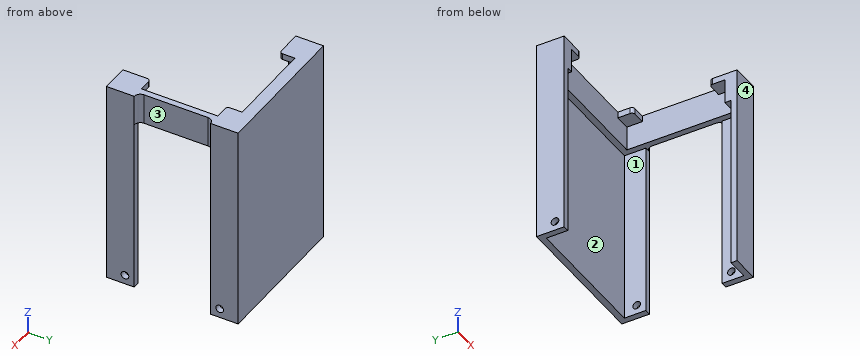
```python
from build123d import *

# Parameters (mm, degrees)
EXTRUDE_THIN1_DEPTH  = 10
SKETCH2_W            = 7
SKETCH2_H            = 7
BOSS_EXTRUDE1_DEPTH  = 2
FILLET1_R            = 1
BOSS_EXTRUDE2_DEPTH  = 67
SKETCH4_R            = 1.25
CUT_EXTRUDE1_DEPTH   = 91.624775862
FILLET2_R            = 2
MOVE_START           = -67
MOVE_FACE1_OUTLINE_W = 29.1
MOVE_FACE1_OUTLINE_H = 2
MOVE_FACE1_DEPTH     = 67


# Read off the part's stored shape, not the designer's step: Move Face1
with BuildPart() as part:
    # Sketch1 → Extrude-Thin1 (new body)
    with BuildSketch(Plane.XY):
        Polygon((0, -5), (0, 0), (39.1, 0), (39.1, -34.8), (34.1, -34.8), (34.1, -36.8), (41.1, -36.8), (41.1, 2), (-2, 2), (-2, -5), align=None)
    extrude(amount=-EXTRUDE_THIN1_DEPTH)

    # Sketch2 → Boss-Extrude1 (add)
    with BuildSketch(Plane.XY):
        with Locations((1.5, -1.5)):
            Rectangle(SKETCH2_W, SKETCH2_H)
        with Locations((37.6, -1.5)):
            Rectangle(SKETCH2_W, SKETCH2_H)
        with Locations((37.6, -33.3)):
            Rectangle(SKETCH2_W, SKETCH2_H)
    extrude(amount=-BOSS_EXTRUDE1_DEPTH)

    # Fillet1
    fillet1_edges = [part.edges().sort_by_distance(p)[0] for p in [
        (5, -5, -1),
        (34.1, -5, -1),
        (34.1, -29.8, -1),
    ]]
    fillet(fillet1_edges, radius=FILLET1_R)

    # Sketch3 → Boss-Extrude2 (add)
    with BuildSketch(Plane.XY):
        Polygon((34.1, 2), (41.1, 2), (41.1, -5), (43.1, -5), (43.1, 4), (34.1, 4), align=None)
    boss_extrude2 = extrude(amount=-BOSS_EXTRUDE2_DEPTH)

    # Mirror1: Boss-Extrude2 across plane
    add(boss_extrude2.mirror(Plane(origin=(19.55, 0, 0), x_dir=(0, 0, 1), z_dir=(1, 0, 0))))

    # Mirror2: Boss-Extrude2 across plane
    add(boss_extrude2.mirror(Plane.ZX.offset(-17.4)))

    # Sketch4 → Cut-Extrude1 (cut, through all)
    with BuildSketch(Plane(origin=(43.1, 0, 0), x_dir=(0, 0, -1), z_dir=(1, 0, 0))):
        with Locations((64, -2)):
            Circle(SKETCH4_R)
    cut_extrude1 = extrude(amount=-CUT_EXTRUDE1_DEPTH, mode=Mode.SUBTRACT)

    # Mirror3: Cut-Extrude1 across plane
    add(cut_extrude1.mirror(Plane.ZX.offset(-17.4)), mode=Mode.SUBTRACT)

    # Fillet2
    fillet2_edges = [part.edges().sort_by_distance(p)[0] for p in [
        (41.1, -29.8, -5),
        (41.1, -5, -5),
    ]]
    fillet(fillet2_edges, radius=FILLET2_R - 0.0001)  # a hair under: the kernel refuses the full size

    # Move Face1 outline → Move Face1 (add)
    with BuildSketch(Plane.XY.offset(MOVE_START)):
        with Locations((19.55, 3)):
            Rectangle(MOVE_FACE1_OUTLINE_W, MOVE_FACE1_OUTLINE_H)
    extrude(amount=MOVE_FACE1_DEPTH)


solid = part.part
```
Design review of the part built by this model. Coordinates are the model's own, in mm. Face numbers are marked on the shaded views. Give positions to 0.01 mm unless a question says otherwise; leave off trailing zeros. Write each loop counter-clockwise with the first axis right and the second up, starting at its lowest first coordinate (ties: lowest second). Pieces come first, ordered by that corner, then holes.
(1) Add section C-C (z = -64). Give the boundary of the cut face in (x, y).
Checked values:
outline: (-4, -5) - (-2, -5) - (-2, -3.25) - (-4, -3.25) - close; (-4, -0.75) - (-2, -0.75) - (-2, 2) - (41.1, 2) - (41.1, -0.75) - (43.1, -0.75) - (43.1, 4) - (-4, 4) - close; (34.1, -38.8) - (43.1, -38.8) - (43.1, -34.05) - (41.1, -34.05) - (41.1, -36.8) - (34.1, -36.8) - close; (41.1, -31.55) - (43.1, -31.55) - (43.1, -29.8) - (41.1, -29.8) - close; (41.1, -5) - (43.1, -5) - (43.1, -3.25) - (41.1, -3.25) - close
(2) Clearance check with flat-ended pins moving along their axes: pin 1 Ø3 at (x, y) = (27.5, -1) entering from +Z; pin 2 Ø1.5 at (x, y) = (2.5, -1.5) entering from -Z; pin 3 Ø9 at (x, z) = (1, -49.5) entering from -Y; pin 4 Ø11 at (y, z) = (-13.5, -6.5) entering from -X. State where each tip first meets the part, or that it passes through.
Checked values:
pin 1: stops at z = 0
pin 2: stops at z = -2
pin 3: stops at y = -5
pin 4: stops at x = 39.1
(3) Add section D-D (z = -37.5). Give the boundary of the cut face in (x, y), and give its area (3 significant figures).
Checked values:
outline: (-4, -5) - (-2, -5) - (-2, 2) - (41.1, 2) - (41.1, -5) - (43.1, -5) - (43.1, 4) - (-4, 4) - close; (34.1, -38.8) - (43.1, -38.8) - (43.1, -29.8) - (41.1, -29.8) - (41.1, -36.8) - (34.1, -36.8) - close
area: 154 mm2
(4) Mouldability with a two-part tool opening along X and no side actions: class the marked faces 1, 2, 3 and 4 as +X half, -X half, draft (parallel to the pull), parting line (faces both ways), or undercut.
Checked values:
face 1: undercut
face 2: undercut
face 3: +X half
face 4: draft
(5) Add section B-B (y = -2). Give the boundary of the cut face in (x, z), and give its area (3 significant figures).
Checked values:
outline: (-4, -67) - (-2, -67) - (-2, -65.25) - (-4, -65.25) - close; (-4, -62.75) - (-2, -62.75) - (-2, -10) - (0, -10) - (0, -2) - (5, -2) - (5, 0) - (-4, 0) - close; (34.1, -2) - (39.1, -2) - (39.1, -10) - (41.1, -10) - (41.1, -62.75) - (43.1, -62.75) - (43.1, 0) - (34.1, 0) - close; (41.1, -67) - (43.1, -67) - (43.1, -65.25) - (41.1, -65.25) - close
area: 318 mm2
(6) Wall thickness on line 1 along Y through (x, z) = (42, -64); line 2 along Y through (x, z) = (41, -64); line 3 along Y through (x, z) = (-3.05, -64): over which ranges is each line inside the solid? List them lowest first.
Checked values:
line 1: y = -38.8 to -34.05, -31.55 to -29.8, -5 to -3.25, -0.75 to 4
line 2: y = -38.8 to -36.8, 2 to 4
line 3: y = -5 to -3.25, -0.75 to 4
(7) Add section A-A (y = -32.8). Give the boundary of the cut face in (x, z), and give its area (3 significant figures).
Checked values:
outline: (34.1, -2) - (39.1, -2) - (39.1, -10) - (41.1, -10) - (41.1, -62.75) - (43.1, -62.75) - (43.1, 0) - (34.1, 0) - close; (41.1, -67) - (43.1, -67) - (43.1, -65.25) - (41.1, -65.25) - close
area: 159 mm2
